```python
from build123d import *

# Parameters (mm, degrees)
SKETCH1_W               = 31.75
SKETCH1_H               = 25.4
BOSS_EXTRUDE1_DEPTH     = 12.7
SKETCH2_W               = 18.25625
SKETCH2_H               = 6.35
CUT_EXTRUDE3_DEPTH      = 39.058949894
SKETCH4_W               = 1.5875
SKETCH4_H               = 4.7625
BOSS_EXTRUDE2_DEPTH     = 31.75
CUT_EXTRUDE5_DEPTH      = 31.590858593
CUT_EXTRUDE5_DEPTH_BACK = 31.590858593
SKETCH5_R               = 0.9921875
CUT_EXTRUDE6_DEPTH      = 1.5875
SKETCH7_R               = 1.984375
CUT_EXTRUDE7_DEPTH      = 1.5875
SKETCH8_W               = 50.8
SKETCH8_H               = 38.305926372
SKETCH8_W_2             = 31.75
SKETCH8_H_2             = 25.4
BOSS_EXTRUDE3_DEPTH     = 3.175
SKETCH10_W              = 31.75
SKETCH10_H              = 3.175
CUT_EXTRUDE8_DEPTH      = 42.677098196
FILLET6_R               = 12.7
CHAMFER1_SIZE           = 1.016
CHAMFER2_SIZE           = 1.524
FILLET7_R               = 3.556
FILLET10_R              = 1.5875


# Some blends are built 0.0001 mm under size
with BuildPart() as part:
    # Sketch1 → Boss-Extrude1 (new body)
    with BuildSketch(Plane(origin=(0, 0, 0), x_dir=(1, 0, 0), z_dir=(0, 1, 0))):
        with Locations((7.914574134, 4.007219009)):
            Rectangle(SKETCH1_W, SKETCH1_H)
    extrude(amount=BOSS_EXTRUDE1_DEPTH)

    # Sketch2 → Cut-Extrude3 (cut, through all)
    with BuildSketch(Plane(origin=(23.789574134, 0, 0), x_dir=(0, 0, -1), z_dir=(1, 0, 0))):
        with Locations((4.007219009, 6.35)):
            Rectangle(SKETCH2_W, SKETCH2_H)
    extrude(amount=-CUT_EXTRUDE3_DEPTH, mode=Mode.SUBTRACT)

    # Sketch4 → Boss-Extrude2 (add, through all)
    with BuildSketch(Plane(origin=(23.789574134, 0, 0), x_dir=(0, 0, -1), z_dir=(1, 0, 0))):
        with Locations((-4.327155991, 7.14375)):
            Rectangle(SKETCH4_W, SKETCH4_H)
        with Locations((12.341594009, 7.14375)):
            Rectangle(SKETCH4_W, SKETCH4_H)
    extrude(amount=-BOSS_EXTRUDE2_DEPTH)

    # Sketch5 → Cut-Extrude5 (cut, two sides: drawn at the far end of the back side and taken through both)
    with BuildSketch(Plane(origin=(0, 3.175, 0), x_dir=(1, 0, 0), z_dir=(0, 1, 0)).offset(-CUT_EXTRUDE5_DEPTH_BACK)):
        with Locations(Location((-2.404175866, 10.754094009, 0), (0, 0, 270))):
            Circle(SKETCH5_R)
        with Locations(Location((18.233324134, 10.754094009, 0), (0, 0, 126.869897646))):
            Circle(SKETCH5_R)
    extrude(amount=CUT_EXTRUDE5_DEPTH + CUT_EXTRUDE5_DEPTH_BACK, mode=Mode.SUBTRACT)

    # Sketch6 → Cut-Extrude6 (cut)
    with BuildSketch(Plane.XZ):
        Polygon((-0.022925866, -10.754094009), (-1.213550866, -8.691871016), (-3.594800866, -8.691871016), (-4.785425866, -10.754094009), (-3.594800866, -12.816317002), (-1.213550866, -12.816317002), align=None)
        Polygon((20.614574134, -10.754094009), (19.423949134, -8.691871016), (17.042699134, -8.691871016), (15.852074134, -10.754094009), (17.042699134, -12.816317002), (19.423949134, -12.816317002), align=None)
    extrude(amount=-CUT_EXTRUDE6_DEPTH, mode=Mode.SUBTRACT)

    # Sketch7 → Cut-Extrude7 (cut)
    with BuildSketch(Plane(origin=(0, 12.7, 0), x_dir=(1, 0, 0), z_dir=(0, 1, 0))):
        with Locations(Location((-2.404175866, 10.754094009, 0), (0, 0, 270))):
            Circle(SKETCH7_R)
        with Locations(Location((18.233324134, 10.754094009, 0), (0, 0, 270))):
            Circle(SKETCH7_R)
    extrude(amount=-CUT_EXTRUDE7_DEPTH, mode=Mode.SUBTRACT)

    # Sketch8 → Boss-Extrude3 (add)
    with BuildSketch(Plane.XZ):
        with Locations((7.914574134, -4.007219009)):
            Rectangle(SKETCH8_W, SKETCH8_H)
        with Locations((7.914574134, -4.007219009)):
            Rectangle(SKETCH8_W_2, SKETCH8_H_2, mode=Mode.SUBTRACT)
    extrude(amount=-BOSS_EXTRUDE3_DEPTH)

    # Sketch10 → Cut-Extrude8 (cut, through all)
    with BuildSketch(Plane(origin=(0, 3.175, 0), x_dir=(1, 0, 0), z_dir=(0, 1, 0))):
        with Locations((7.914574134, 18.294719009)):
            Rectangle(SKETCH10_W, SKETCH10_H)
        with Locations((7.914574134, -10.280280991)):
            Rectangle(SKETCH10_W, SKETCH10_H)
    extrude(amount=-CUT_EXTRUDE8_DEPTH, mode=Mode.SUBTRACT)

    # Fillet6
    fillet6_edges = [part.edges().sort_by_distance(p)[0] for p in [
        (-17.485425866, 1.5875, 15.145744177),
        (33.314574134, 1.5875, 15.145744177),
        (33.314574134, 1.5875, -23.160182195),
        (-17.485425866, 1.5875, -23.160182195),
    ]]
    fillet(fillet6_edges, radius=FILLET6_R)

    # Chamfer1
    # the kernel refuses this chamfer: 1.016 mm, written as the material it takes off along each edge
    with BuildSketch(Plane(origin=(-7.960425866, 4.7625, 0.920576075), x_dir=(-0.027495876610586435, 0.9996219169112968, 0), z_dir=(0, 0, 1)), Plane(origin=(-7.960425866, 4.7625, -13.135344009), x_dir=(-0.027495876610586435, 0.9996219169112968, 1.1185418764848949e-15), z_dir=(0, 0, 1))) as chamfer1_piece_1:
        Polygon((CHAMFER1_SIZE * 0.999621916911, -CHAMFER1_SIZE * 0.0274958766106), (-CHAMFER1_SIZE * 0.0274958766106, -CHAMFER1_SIZE * 0.999621916911), (0, 0), align=None)
    extrude(amount=4.200329916, mode=Mode.SUBTRACT)
    with BuildSketch(Plane(origin=(26.402404049, 4.7625, 3.533405991), x_dir=(0, 0.9996219169112968, -0.027495876610586435), z_dir=(-1, 0, 0))) as chamfer1_piece_2:
        Polygon((CHAMFER1_SIZE * 0.999621916911, -CHAMFER1_SIZE * 0.0274958766106), (-CHAMFER1_SIZE * 0.0274958766106, -CHAMFER1_SIZE * 0.999621916911), (0, 0), align=None)
    extrude(amount=36.975659832, mode=Mode.SUBTRACT)
    with BuildSketch(Plane(origin=(23.789574134, 4.7625, 0.920576075), x_dir=(0.027495876610587285, 0.9996219169112968, 0), z_dir=(0, 0, 1)), Plane(origin=(23.789574134, 4.7625, -13.135344009), x_dir=(0.027495876610587285, 0.9996219169112968, 1.1185418764848949e-15), z_dir=(0, 0, 1))) as chamfer1_piece_3:
        Polygon((CHAMFER1_SIZE * 0.999621916911, CHAMFER1_SIZE * 0.0274958766106), (-CHAMFER1_SIZE * 0.0274958766106, CHAMFER1_SIZE * 0.999621916911), (0, 0), align=None)
    extrude(amount=4.200329916, mode=Mode.SUBTRACT)
    with BuildSketch(Plane(origin=(-0.386658451, 4.7625, -11.547844009), x_dir=(0, -0.027495876610585605, -0.9996219169112968), z_dir=(-1, 0, 0)), Plane(origin=(26.402404049, 4.7625, -11.547844009), x_dir=(0, -0.027495876610585605, -0.9996219169112968), z_dir=(-1, 0, 0))) as chamfer1_piece_4:
        Polygon((CHAMFER1_SIZE * 0.999621916911, -CHAMFER1_SIZE * 0.0274958766106), (-CHAMFER1_SIZE * 0.0274958766106, -CHAMFER1_SIZE * 0.999621916911), (0, 0), align=None)
    extrude(amount=10.186597332, mode=Mode.SUBTRACT)
    with BuildSketch(Plane(origin=(20.250841549, 4.7625, -11.547844009), x_dir=(0, -0.027495876610585605, -0.9996219169112968), z_dir=(-1, 0, 0))) as chamfer1_piece_5:
        Polygon((CHAMFER1_SIZE * 0.999621916911, -CHAMFER1_SIZE * 0.0274958766106), (-CHAMFER1_SIZE * 0.0274958766106, -CHAMFER1_SIZE * 0.999621916911), (0, 0), align=None)
    extrude(amount=24.672534832, mode=Mode.SUBTRACT)

    # Chamfer2
    chamfer2_edges = [part.edges().sort_by_distance(p)[0] for p in [
        (-7.960425866, 7.65175, 3.533405991),
        (23.789574134, 7.65175, 3.533405991),
        (-7.960425866, 7.65175, -11.547844009),
        (23.789574134, 7.65175, -11.547844009),
    ]]
    chamfer(chamfer2_edges, length=CHAMFER2_SIZE)

    # Fillet7
    # the kernel refuses this fillet: 3.556 mm, written as the material it takes off along each edge
    with BuildSketch(Plane(origin=(20.233574134, 9.144, 5.136780991), x_dir=(0, 0, 1), z_dir=(1, 0, 0))) as fillet7_piece_1_section:
        Polygon((0, 0), (FILLET7_R * 1.02, 0), (FILLET7_R * 1.02, -FILLET7_R * 1.02), (0, -FILLET7_R * 1.02), align=None)
    fillet7_piece_1 = extrude(amount=FILLET7_R * 1.02, mode=Mode.PRIVATE)
    fillet7_piece_1 = fillet7_piece_1 - Plane(origin=(20.233574134, 9.144, 5.136780991), x_dir=(0, -0.7071067811865475, -0.7071067811865475), z_dir=(1, 0, 0)) * Sphere(FILLET7_R, mode=Mode.PRIVATE)
    add(fillet7_piece_1, mode=Mode.SUBTRACT)
    with BuildSketch(Plane(origin=(-4.404425866, 9.144, 5.136780991), x_dir=(0, 0, 1), z_dir=(-1, 0, 0))) as fillet7_piece_2_section:
        Polygon((0, 0), (FILLET7_R * 1.02, 0), (FILLET7_R * 1.02, FILLET7_R * 1.02), (0, FILLET7_R * 1.02), align=None)
    fillet7_piece_2 = extrude(amount=FILLET7_R * 1.02, mode=Mode.PRIVATE)
    fillet7_piece_2 = fillet7_piece_2 - Plane(origin=(-4.404425866, 9.144, 5.136780991), x_dir=(0, -0.7071067811865475, -0.7071067811865475), z_dir=(-1, 0, 0)) * Sphere(FILLET7_R, mode=Mode.PRIVATE)
    add(fillet7_piece_2, mode=Mode.SUBTRACT)
    with BuildSketch(Plane(origin=(20.233574134, 9.144, -13.151219009), x_dir=(1, 0, 0), z_dir=(0, 0, -1))) as fillet7_piece_3_section:
        Polygon((0, 0), (FILLET7_R * 1.02, 0), (FILLET7_R * 1.02, -FILLET7_R * 1.02), (0, -FILLET7_R * 1.02), align=None)
    fillet7_piece_3 = extrude(amount=FILLET7_R * 1.02, mode=Mode.PRIVATE)
    fillet7_piece_3 = fillet7_piece_3 - Plane(origin=(20.233574134, 9.144, -13.151219009), x_dir=(-0.7071067811865475, -0.7071067811865475, 0), z_dir=(0, 0, -1)) * Sphere(FILLET7_R, mode=Mode.PRIVATE)
    add(fillet7_piece_3, mode=Mode.SUBTRACT)
    with BuildSketch(Plane(origin=(-4.404425866, 9.144, -13.151219009), x_dir=(-1, 0, 0), z_dir=(0, 0, -1))) as fillet7_piece_4_section:
        Polygon((0, 0), (FILLET7_R * 1.02, 0), (FILLET7_R * 1.02, FILLET7_R * 1.02), (0, FILLET7_R * 1.02), align=None)
    fillet7_piece_4 = extrude(amount=FILLET7_R * 1.02, mode=Mode.PRIVATE)
    fillet7_piece_4 = fillet7_piece_4 - Plane(origin=(-4.404425866, 9.144, -13.151219009), x_dir=(0.7071067811865475, -0.7071067811865475, 0), z_dir=(0, 0, -1)) * Sphere(FILLET7_R, mode=Mode.PRIVATE)
    add(fillet7_piece_4, mode=Mode.SUBTRACT)
    with BuildSketch(Plane(origin=(20.233574134, 12.7, 8.692780991), x_dir=(0, -1, 0), z_dir=(-1, 0, 0))) as fillet7_piece_5:
        with BuildLine():
            CenterArc((FILLET7_R, -FILLET7_R), FILLET7_R, 90, 90)
            Line((0, -FILLET7_R), (0, 0))
            Line((0, 0), (FILLET7_R, 0))
        make_face()
    extrude(amount=24.638, mode=Mode.SUBTRACT)
    with BuildSketch(Plane(origin=(23.789574134, 3.175, 8.692780991), x_dir=(-1, 0, 0), z_dir=(0, 1, 0)), Plane(origin=(-7.960425866, 3.175, -16.707219009), x_dir=(1, 0, 0), z_dir=(0, 1, 0))) as fillet7_piece_6:
        with BuildLine():
            CenterArc((FILLET7_R, -FILLET7_R), FILLET7_R, 90, 90)
            Line((0, -FILLET7_R), (0, 0))
            Line((0, 0), (FILLET7_R, 0))
        make_face()
    extrude(amount=5.969, mode=Mode.SUBTRACT)
    with BuildSketch(Plane(origin=(23.789574134, 12.7, -13.151219009), x_dir=(-1, 0, 0), z_dir=(0, 0, 1)), Plane(origin=(-7.960425866, 12.7, 5.136780991), x_dir=(1, 0, 0), z_dir=(0, 0, -1))) as fillet7_piece_7:
        with BuildLine():
            CenterArc((FILLET7_R, FILLET7_R), FILLET7_R, 180, 90)
            Line((0, FILLET7_R), (0, 0))
            Line((0, 0), (FILLET7_R, 0))
        make_face()
    extrude(amount=18.288, mode=Mode.SUBTRACT)
    with BuildSketch(Plane(origin=(23.789574134, 3.175, -16.707219009), x_dir=(-1, 0, 0), z_dir=(0, 1, 0)), Plane(origin=(-7.960425866, 3.175, 8.692780991), x_dir=(1, 0, 0), z_dir=(0, 1, 0))) as fillet7_piece_8:
        with BuildLine():
            CenterArc((FILLET7_R, FILLET7_R), FILLET7_R, 180, 90)
            Line((0, FILLET7_R), (0, 0))
            Line((0, 0), (FILLET7_R, 0))
        make_face()
    extrude(amount=5.969, mode=Mode.SUBTRACT)
    with BuildSketch(Plane(origin=(-4.404425866, 12.7, -16.707219009), x_dir=(0, 0, 1), z_dir=(1, 0, 0))) as fillet7_piece_9:
        with BuildLine():
            CenterArc((FILLET7_R, FILLET7_R), FILLET7_R, 180, 90)
            Line((0, FILLET7_R), (0, 0))
            Line((0, 0), (FILLET7_R, 0))
        make_face()
    extrude(amount=24.638, mode=Mode.SUBTRACT)

    # Fillet10
    fillet10_edges = [part.edges().sort_by_distance(p)[0] for p in [
        (7.914574134, 3.175, 15.145744177),
        (7.914574134, 0, 15.145744177),
        (-17.485425866, 0, -4.007219009),
        (7.914574134, 0, -23.160182195),
        (33.314574134, 0, -4.007219009),
        (29.594830255, 0, 11.426000298),
        (29.594830255, 0, -19.440438316),
        (-13.765681988, 0, -19.440438316),
        (-13.765681988, 0, 11.426000298),
        (-17.485425866, 3.175, -4.007219009),
        (33.314574134, 3.175, -4.007219009),
        (7.914574134, 3.175, -23.160182195),
    ]]
    fillet(fillet10_edges, radius=FILLET10_R - 0.0001)  # a hair under: the kernel refuses the full size


solid = part.part
```
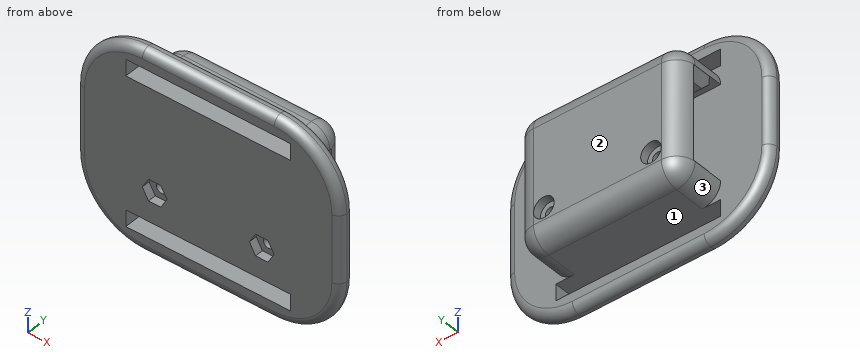
Part model, mm, in its own coordinate system. Face numbers are marked on the shaded views. Give positions to 0.01 mm unless a question says otherwise; leave off trailing zeros. Write each loop counter-clockwise with the first axis right and the second up, starting at its lowest first coordinate (ties: lowest second). Pieces come first, ordered by that corner, then holes. Notation, with made-up numbers: M 32.5,12 L 60.5,12 A14 ccw 60.5,21 Z; hole C 63.25,7 d7. An arc over 180 degrees is marked long. Use CSV: the item, a comma, the result in double quotes.
Item 1: Drill centre lines: probe 1 along Y at (x, z) = (-3.5, -3.5) (3 decimals); probe 2 along X at (y, z) = (10.5, -10); probe 3 along Z at (x, y) = (13, 7.25). Where is each one in solid material? Low to high.
Taken from the geometry:
probe 1,"y = 0 to 3.175, 9.525 to 12.7"
probe 2,"x = -7.69 to -3.05, -1.76 to 17.59, 18.88 to 23.52"
probe 3,"z = -16.71 to -11.55, 3.53 to 8.69"
Item 2: Slice it at A-A on x = 3. State how many separate pieces and enclosed holes the cut face has, plus the area to 3 significant figures.
Taken from the geometry:
separate pieces,"3"
enclosed holes,"1"
area,"234 mm²"
Item 3: Slice it at B-B on y = 6.5. Write the cut outline in (x, z).
Taken from the geometry:
outline,"M -7.96,-13.15 A3.56 ccw -4.4,-16.71 L 20.23,-16.71 A3.56 ccw 23.79,-13.15 L 23.79,-13.07 L 22.27,-11.55 L 18.83,-11.55 A0.99 cw 17.64,-11.55 L -1.81,-11.55 A0.99 cw -3,-11.55 L -6.44,-11.55 L -7.96,-13.07 Z; M -7.96,5.06 L -6.44,3.53 L 22.27,3.53 L 23.79,5.06 L 23.79,5.14 A3.56 ccw 20.23,8.69 L -4.4,8.69 A3.56 ccw -7.96,5.14 Z"
Item 4: Pin check, flat tips, straight feed: P1, Ø1, axis at y = 1, z = 10.5, coming from the -X side; P2, Ø3, axis at y = 9, z = -16.5, coming from the +X side; P3, Ø3, axis at x = 18.23, z = -10.75, coming from the -Y side; P4, Ø4.5, axis at x = 18.5, z = -10, coming from the -Y side. Stop position of each tip, or through.
Taken from the geometry:
P1,"stops at x = -14.9"
P2,"stops at x = 23.27"
P3,"stops at y = 1.59"
P4,"stops at y = 0"
Item 5: Pull direction X, two halves, no side cores. Call the marked faces 1, 2 and 3: +X half, -X half, draft (parallel to the pull), parting line (faces both ways), or undercut.
Taken from the geometry:
face 1,"undercut"
face 2,"draft"
face 3,"-X half"
